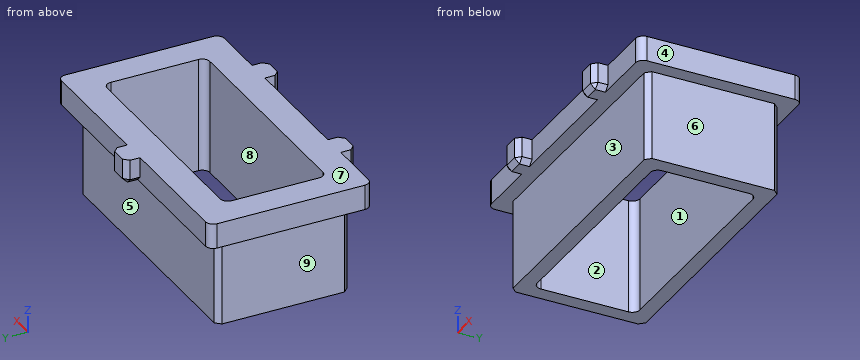
from build123d import *

# Parameters (mm, degrees)
SKETCH1_W           = 13.3985
SKETCH1_H           = 6.731
SKETCH1_W_2         = 11.8745
SKETCH1_H_2         = 5.207
EXTRUDE_THIN1_DEPTH = 5.8039
SKETCH2_W           = 14.9225
SKETCH2_H           = 8.255
SKETCH2_W_2         = 13.3985
SKETCH2_H_2         = 6.731
EXTRUDE_THIN2_DEPTH = 1.27
SKETCH4_W           = 1.27
SKETCH4_H           = 0.762
BOSS_EXTRUDE1_DEPTH = 1.27
CHAMFER1_SIZE       = 0.254
FILLET1_R           = 0.381


with BuildPart() as part:
    # Sketch1 → Extrude-Thin1 (new body)
    with BuildSketch(Plane.XY):
        with Locations((23.121102666, 199.184077883)):
            Rectangle(SKETCH1_W, SKETCH1_H)
        with Locations((23.121102666, 199.184077883)):
            Rectangle(SKETCH1_W_2, SKETCH1_H_2, mode=Mode.SUBTRACT)
    extrude(amount=EXTRUDE_THIN1_DEPTH)

    # Sketch2 → Extrude-Thin2 (add)
    with BuildSketch(Plane.XY.offset(5.8039)):
        with Locations((23.121102666, 199.184077883)):
            Rectangle(SKETCH2_W, SKETCH2_H)
        with Locations((23.121102666, 199.184077883)):
            Rectangle(SKETCH2_W_2, SKETCH2_H_2, mode=Mode.SUBTRACT)
    extrude(amount=-EXTRUDE_THIN2_DEPTH)

    # Sketch4 → Boss-Extrude1 (add)
    with BuildSketch(Plane.XY.offset(5.8039)):
        with Locations((23.121102666, 203.692577883)):
            Rectangle(SKETCH4_W, SKETCH4_H)
        with Locations((26.851727666, 194.675577883)):
            Rectangle(SKETCH4_W, SKETCH4_H)
        with Locations((19.390477666, 194.675577883)):
            Rectangle(SKETCH4_W, SKETCH4_H)
    extrude(amount=-BOSS_EXTRUDE1_DEPTH)

    # Chamfer1
    chamfer1_edges = [part.edges().sort_by_distance(p)[0] for p in [
        (16.421852666, 195.818577883, 2.26695),
        (16.421852666, 202.549577883, 2.26695),
        (29.820352666, 202.549577883, 2.26695),
        (29.820352666, 195.818577883, 2.26695),
        (22.486102666, 203.692577883, 4.5339),
        (23.121102666, 204.073577883, 4.5339),
        (22.486102666, 204.073577883, 5.1689),
        (23.756102666, 203.692577883, 4.5339),
        (23.756102666, 204.073577883, 5.1689),
        (27.486727666, 194.675577883, 4.5339),
        (26.851727666, 194.294577883, 4.5339),
        (27.486727666, 194.294577883, 5.1689),
        (26.216727666, 194.675577883, 4.5339),
        (26.216727666, 194.294577883, 5.1689),
        (20.025477666, 194.675577883, 4.5339),
        (19.390477666, 194.294577883, 4.5339),
        (20.025477666, 194.294577883, 5.1689),
        (18.755477666, 194.675577883, 4.5339),
        (18.755477666, 194.294577883, 5.1689),
    ]]
    chamfer(chamfer1_edges, length=CHAMFER1_SIZE)

    # Fillet1
    fillet1_edges = [part.edges().sort_by_distance(p)[0] for p in [
        (15.659852666, 203.311577883, 5.1689),
        (15.659852666, 195.056577883, 5.1689),
        (30.582352666, 195.056577883, 5.1689),
        (30.582352666, 203.311577883, 5.1689),
        (29.058352666, 201.787577883, 2.90195),
        (17.183852666, 201.787577883, 2.90195),
        (29.058352666, 196.580577883, 2.90195),
        (17.183852666, 196.580577883, 2.90195),
    ]]
    fillet(fillet1_edges, radius=FILLET1_R)


solid = part.part
The listing builds one solid part. Answer for the finished solid, in the listing's coordinates (mm). Face numbers are marked on the shaded views. A direction names the side the tool comes from. Give positions to 0.01 mm unless a question says otherwise; leave off trailing zeros. Write each loop counter-clockwise with the first axis right and the second up, starting at its lowest first coordinate (ties: lowest second). Pieces come first, ordered by that corner, then holes. Notation, with made-up numbers: (77, 44) - (125, 44) arc R16 cw to (125, 60) - close; hole circle Ø2 at (-39.75, 11.25). An arc over 180 degrees is marked (long way). One line per question, with ' | ' between items. Start each with the question number.
1. Determine the mould class of the marked faces 1, 2, 3 and 4 for opening direction Y: +Y half, -Y half, draft (parallel to the pull), parting line (faces both ways), or undercut.
2. Section D-D, the plane y = 196.25 is taken. Determine the outline of the cut face in (x, z), then the cut area to 3 significant figures.
3. For the marked faces 5, 6, 7, 8 and 9, determine the directions among +Z, -Z, +X, -X, +Y, -Y from which every point of the face is accessible in a straight line to the end or side of a thin tool.
4. Section B-B, the plane x = 25 is taken. Determine the outline of the cut face in (y, z), then the cut area to 3 significant figures.
5. Straight lines are drawn through the part: line 1 (Y direction, x = 25.25, z = 3); line 2 (X direction, y = 201.25, z = 1.2); line 3 (Y direction, x = 24.25, z = 5). For each, find the intervals that lie inside material, in ascending order.
6. Given P1, Ø2, axis at x = 28.5, y = 197.5, coming from the -Z side; P2, Ø0.6, axis at x = 18, z = 5, coming from the -Y side; P3, Ø0.6, axis at y = 195, z = 5, coming from the -X side; P4, Ø2, axis at x = 25.5, z = 1, coming from the -Y side, each flat-ended and moving along its own axis, determine where each tip first touches the part or whether it passes through.
7. Section A-A, the plane y = 198.75 is taken. Determine the outline of the cut face in (x, z), then the cut area to 3 significant figures.
Result:
1) face 1: undercut | face 2: undercut | face 3: -Y half | face 4: draft
2) outline: (15.66, 4.53) - (16.42, 4.53) - (16.42, 0) - (29.82, 0) - (29.82, 4.53) - (30.58, 4.53) - (30.58, 5.8) - (15.66, 5.8) - close | area: 79.7 mm2
3) face 5: -Z, +X, -X, +Y | face 6: -Z, +X, +Y, -Y | face 7: +Z, +X, -X, +Y, -Y | face 8: +Z, -Z | face 9: -Z, -X, +Y, -Y
4) outline: (195.06, 4.53) - (195.82, 4.53) - (195.82, 0) - (196.58, 0) - (196.58, 5.8) - (195.06, 5.8) - close; (201.79, 0) - (202.55, 0) - (202.55, 4.53) - (203.31, 4.53) - (203.31, 5.8) - (201.79, 5.8) - close | area: 10.8 mm2
5) line 1: y = 195.82 to 196.58, 201.79 to 202.55 | line 2: x = 16.42 to 17.18, 29.06 to 29.82 | line 3: y = 195.06 to 196.58, 201.79 to 203.31
6) P1: stops at z = 0 | P2: stops at y = 195.06 | P3: stops at x = 15.69 | P4: stops at y = 195.82
7) outline: (15.66, 4.53) - (16.42, 4.53) - (16.42, 0) - (17.18, 0) - (17.18, 5.8) - (15.66, 5.8) - close; (29.06, 0) - (29.82, 0) - (29.82, 4.53) - (30.58, 4.53) - (30.58, 5.8) - (29.06, 5.8) - close | area: 10.8 mm2
